Geometry check sheet. Reference: drawing and pictorial views, mm from the part's lowest x, y, z. A direction names the side the tool comes from. Round coordinates to 2 decimals unless told otherwise and drop trailing zeros. Order: outer loops, then holes, each group sorted by start corner. A loop starts at its lowest first (then second) coordinate and runs counter-clockwise, first axis right, second up.
(1) Depth check by flat-ended pin: pin 1 (1 mm diameter, centred on x = 7, y = 7.5, fed in from -Z); pin 2 (1.5 mm diameter, centred on y = 8.5, z = 12, fed in from +X); pin 3 (3 mm diameter, centred on y = 7, z = 10.5, fed in from -X). Enter the tip coordinate at first touch or a pass-through.
(2) Sectioned sample at D-D, the plane z = 12.25. Enter the section's corners in (x, y).
(3) Tool access check on the marked faces 1 and 2. Record the directions out of +Z, -Z, +X, -X, +Y, -Y that give a thin tool (end or side, any length) a straight path to the whole face; none if there is none.
(4) Thickness scan on probe 1 along Y at (x, z) = (1, 8.25); probe 2 along Z at (x, y) = (10, 8); probe 3 along Z at (x, y) = (9, 9). Record the ranges inside material, lowest first.
(5) Sectioned sample at C-C, the plane y = 7.75. Enter the section's corners in (x, z).
(6) Sectioned sample at A-A, the plane x = 7. Enter the section's corners in (y, z), and give its area (3 significant figures).
(7) Sectioned sample at B-B, the plane z = 7. Enter the section's corners in (x, y), and give its area (3 significant figures).
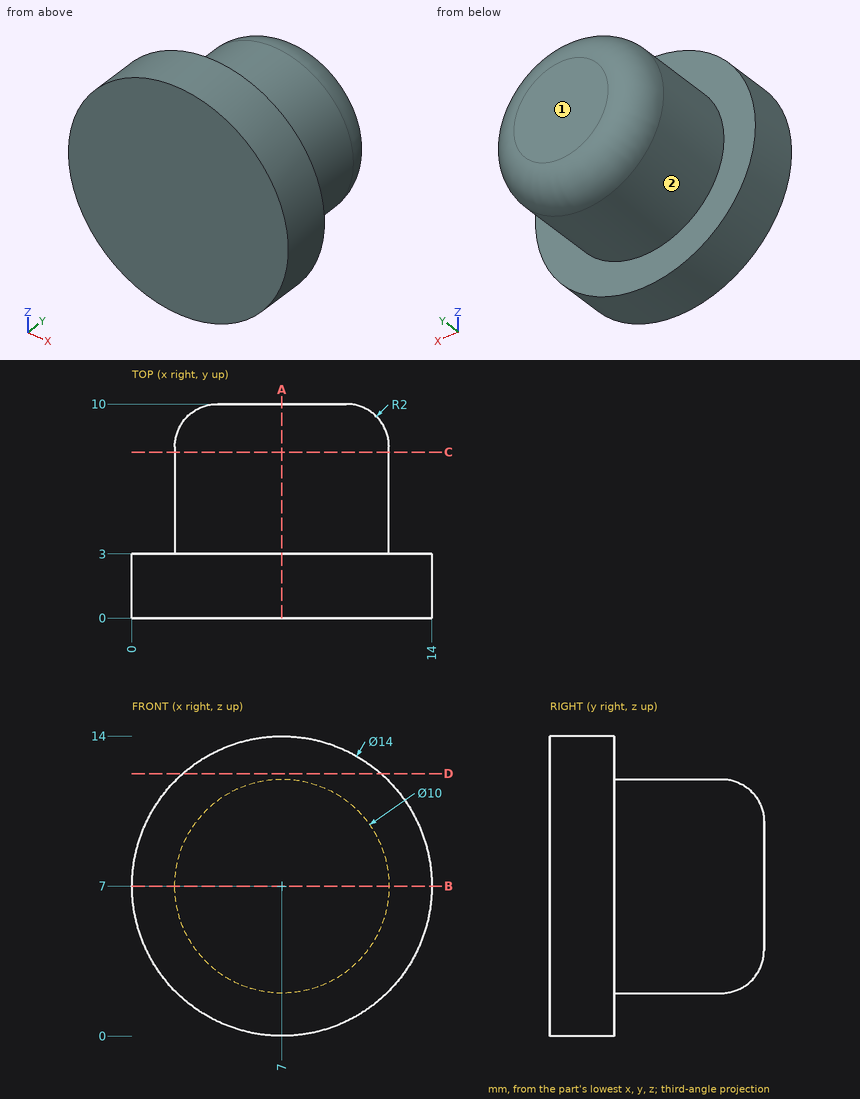
Derived:
1. pin 1: stops at z = 2
1. pin 2: stops at x = 9.55
1. pin 3: stops at x = 2.42
2. outline: (2.37, 0) - (11.63, 0) - (11.63, 3) - (2.37, 3) - close
3. face 1: +Z, -Z, +X, -X, +Y
3. face 2: +Y
4. probe 1: y = 0 to 3
4. probe 2: z = 3 to 11
4. probe 3: z = 2.71 to 11.29
5. outline: circle Ø10 at (7, 7)
6. outline: (0, 0) - (3, 0) - (3, 2) - (8, 2) arc R2 ccw to (10, 4) - (10, 10) arc R2 ccw to (8, 12) - (3, 12) - (3, 14) - (0, 14) - close
6. area: 110 mm2
7. outline: (0, 0) - (14, 0) - (14, 3) - (12, 3) - (12, 8) arc R2 ccw to (10, 10) - (4, 10) arc R2 ccw to (2, 8) - (2, 3) - (0, 3) - close
7. area: 110 mm2
